Can you work these out from the model? Positions are in its coordinate system, mm. A direction names the side the tool comes from. Give positions to 0.01 mm unless a question says otherwise; leave off trailing zeros. Order: outer loops, then holes, each group sorted by start corner. A loop starts at its lowest first (then second) coordinate and runs counter-clockwise, first axis right, second up. Notation, with made-up numbers: M 47,-36.5 L 83,-36.5 A18 ccw 83,-19.5 Z; hole C 77,31.25 d11. An arc over 180 degrees is marked long. Write each question's results on one line, items separated by ' | '.
from build123d import *

# Parameters (mm, degrees)
F1_DEPTH      = 77.47
F3_DEPTH      = 1.27
F5_W          = 74.93
F5_H          = 87.551641
F5_W_2        = 72.39
F5_H_2        = 85.011641
F6_DEPTH      = 3.175
F6_DEPTH_BACK = 1.27
F7_W          = 74.93
F7_H          = 24.13
F8_DEPTH      = 9.5758
F10_W         = 74.93
F10_H         = 24.13
F10_W_2       = 70.358
F10_H_2       = 19.558
F11_DEPTH     = 1.905


# Not quite as in the source:
# - a pattern or mirror of a feature is missing from the dataset's text; its kind, count and spacing are read off the source's solid


with BuildPart() as f1:
    # F0 (on Right) → F1 (new body)
    with BuildSketch(Plane.YZ):
        Polygon((88.9000101356, 0), (90.1700101356, 0), (90.1700101356, 6.0914319939), (72.2094978935, 24.0519442361), (0, 4.7625), (0, 0), (1.3483691356, 0), (1.3483691356, 3.8081596938), (71.8294909699, 22.6358999354), (88.9000101356, 5.5653807697), align=None)
    extrude(amount=F1_DEPTH)

    # F2 (on face) → F3 (join)
    with BuildSketch(Plane.YZ.offset(77.47)):
        Polygon((0, 0), (90.1700101356, 0), (90.1700101356, 6.0914319939), (72.2094978935, 24.0519442361), (0, 4.7625), align=None)
    f3 = extrude(amount=-F3_DEPTH)

    # F3_copies: F3 across plane
    add(f3.mirror(Plane(origin=(38.735, 0, 0), x_dir=(0, 0, -1), z_dir=(-1, 0, 0))))

    # F5 (on face) → F6 (join, two sides)
    with BuildSketch(Plane(origin=(0, 0, 0), x_dir=(1, 0, 0), z_dir=(0, 0, -1))) as f6_sk:
        with Locations((38.735, -45.1241896356)):
            Rectangle(F5_W, F5_H)
        with Locations((38.735, -45.1241896356)):
            Rectangle(F5_W_2, F5_H_2, mode=Mode.SUBTRACT)
    extrude(amount=F6_DEPTH)
    extrude(f6_sk.sketch, amount=-F6_DEPTH_BACK)

    # F7 (on face) → F8 (cut)
    with BuildSketch(Plane(origin=(0, 48.1307210648, 48.1307210648), x_dir=(1, 0, 0), z_dir=(0, 0.7071067812, 0.7071067812))):
        with Locations((38.735, 46.7525327565)):
            Rectangle(F7_W, F7_H)
    extrude(amount=-F8_DEPTH, mode=Mode.SUBTRACT)

    # F10 (on offset) → F11 (join)
    with BuildSketch(Plane(origin=(0, 41.3596079495, 41.3596079495), x_dir=(1, 0, 0), z_dir=(0, 0.7071067812, 0.7071067812))):
        with Locations((38.735, 46.7525327565)):
            Rectangle(F10_W, F10_H)
        with Locations((38.735, 46.7525327565)):
            Rectangle(F10_W_2, F10_H_2, mode=Mode.SUBTRACT)
    extrude(amount=-F11_DEPTH)


solid = f1.part
(1) Imagine slicing it at A-A, the plane x = 16.5. Count the separate pieces of the cut face and the enclosed holes in it, plus the area to 3 significant figures.
Data:
separate pieces: 4 | enclosed holes: 0 | area: 128 mm2
(2) I need wall thicknesses on L1, parallel to Y at x = 61, z = 2.75; L2, parallel to X at y = 25, z = 10; L3, parallel to Y at x = 61.5, z = -1. Which ranges of each line are inside material? Lowest first, please. Write a range as from..to.
Data:
L1: y = 0..1.35, 88.9..90.17 | L2: x = 0..1.27, 76.2..77.47 | L3: y = 1.35..2.62, 81.03..82.18, 87.63..88.9
(3) For faces 4 (the face through (38, 87.63, -1)), 5 (the face through (1.27, 46, -2)), 6 (the face through (2, 23, 1.27)), 7 (the face through (38, 1.348, -2)), 8 (the face through (2.54, 46, -1)), which set-ups out of +Z, -Z, +X, -X, +Y, -Y let a thin tool reach every point of the face, with its end or its side?
Data:
face 4: +Z, -Z | face 5: -Z, -X, +Y, -Y | face 6: none | face 7: -Z, +X, -X, -Y | face 8: -Z
(4) Imagine slicing it at C-C, the plane z = 11. Write out the boundary of the cut face in (x, y).
Data:
outline: M 0,23.35 L 77.47,23.35 L 77.47,85.26 L 76.2,85.26 L 76.2,71.72 L 73.91,71.72 L 73.91,69.03 L 76.2,69.03 L 76.2,28.27 L 1.27,28.27 L 1.27,69.03 L 3.56,69.03 L 3.56,71.72 L 1.27,71.72 L 1.27,85.26 L 0,85.26 Z
(5) Imagine slicing it at D-D, the plane z = 18. Write out the boundary of the cut face in (x, y).
Data:
outline: M 0,49.55 L 77.47,49.55 L 77.47,78.26 L 76.2,78.26 L 76.2,54.48 L 1.27,54.48 L 1.27,78.26 L 0,78.26 Z
(6) Imagine slicing it at B-B, the plane y = 60. Write out the boundary of the cut face in (x, z) (3 decimals), plus the area to 3 significant figures.
Data:
outline: M 0,0 L 1.27,0 L 1.27,-3.175 L 2.54,-3.175 L 2.54,1.27 L 1.27,1.27 L 1.27,19.476 L 76.2,19.476 L 76.2,1.27 L 74.93,1.27 L 74.93,-3.175 L 76.2,-3.175 L 76.2,0 L 77.47,0 L 77.47,20.79 L 0,20.79 Z | area: 163 mm2
(7) Will these pins go through, and if not, where does the flat tip stop? P1, Ø4, axis at x = 44.5, y = 24.5, coming from the +Z side; P2, Ø4, axis at x = 15, z = 8.5, coming from the +Y side; P3, Ø1, axis at y = 30.5, z = -1, coming from the -X side.
Data:
P1: stops at z = 11.84 | P2: stops at y = 89.76 | P3: stops at x = 1.27
(8) We'd pull the mould along Z, two halves only. Please class faces 1 (the face through (38.193, 36.61, 14.542)), 2 (the face through (38, 0, 2)), 3 (the face through (1.27, 55, 9)): +Z half, -Z half, draft (parallel to the pull), parting line (faces both ways), or undercut.
Data:
face 1: +Z half | face 2: draft | face 3: undercut
